CAD build for the part. Positions are in the model's coordinates, mm. Give positions to 0.01 mm unless a question says otherwise; leave off trailing zeros. Loops run counter-clockwise (first coordinate to the right, second up) from the corner with the lowest first, then second, coordinate; pieces in that order, holes last.
Item 1: Saw through at D-D on z = 5.5. Give the cut face in (x, y).
Item 2: Mould opens along X. For faces 1 (the flat face through (0, 0, -12)), 2 (the flat face through (-9.525, 2, -13)), 3 (the cylindrical face through (0.28, 1.9, -27.54)) say: released by +X, released by -X, zero draft, split by the parting line, or undercut.
Item 3: Saw through at C-C on z = 1. Give the cut face in (x, y), plus the area to 3 significant figures.
Item 4: Saw through at B-B on y = 2.95. Give the cut face in (x, z) (3 decimals), plus the area to 3 significant figures.
Item 5: Probe probe 1 along Z at (x, y) = (0, 1) (3 decimals); probe 2 along X at (y, z) = (2.75, -25) (3 decimals); probe 3 along X at (y, z) = (0.65, -1.5) (3 decimals). List the from-to ranges inside material, lowest first.
Item 6: Saw through at A-A on x = 0. Give the cut face in (y, z) (3 decimals), plus the area to 3 significant figures.
Item 7: Drop flat-ended pins along their axis: P1, Ø3.5, axis at x = 0, z = -25.4, coming from the +Y side; P2, Ø8, axis at x = -1.5, z = -19, coming from the -Y side. Give the stop position or say it passes through.
Autodesk Inventor part; units mm, degrees
ref_plane "YZ Plane" through (0, 0, 0) normal (1, 0, 0) x (0, 1, 0)
ref_plane "XZ Plane" through (0, 0, 0) normal (0, 1, 0) x (-1, 0, 0)
ref_plane "XY Plane" through (0, 0, 0) normal (0, 0, 1) x (1, 0, 0)
sketch "Sketch1" plane through (0, 0, 0) normal (0, 1, 0) x (-1, 0, 0)
  circle A0 centre (0, 0) radius 2.159
  circle A1 centre (0, -25.4) radius 2.159
  line L0 (0, 0) -> (0, -25.4) construction
  line L1 (-9.525, 0) -> (-9.525, -25.4)
  line L2 (9.525, -25.4) -> (9.525, 0)
  arc A2 (9.525, 0) -> (-9.525, 0) centre (0, 0) ccw
  arc A3 (-9.525, -25.4) -> (9.525, -25.4) centre (0, -25.4) ccw
  point P0 (0, -12.7)
  dimension "d0" = 4.318
  dimension "d2" = 25.4
  dimension "d3" = 19.05
extrude "Extrusion1" add sketch "Sketch1" along normal blind 3.861
properties part number "Small Motor Spacer" material "PET Plastic"
Results below:
1. outline: (-7.78, 0) - (7.78, 0) - (7.78, 3.86) - (-7.78, 3.86) - close
2. face 1: zero draft
2. face 2: released by -X
2. face 3: undercut
3. outline: (-9.47, 0) - (-1.91, 0) - (-1.91, 3.86) - (-9.47, 3.86) - close; (1.91, 0) - (9.47, 0) - (9.47, 3.86) - (1.91, 3.86) - close
3. area: 58.4 mm2
4. outline: (-9.525, -25.4) arc R9.525 ccw to (9.525, -25.4) - (9.525, 0) arc R9.525 ccw to (-9.525, 0) - close; hole circle Ø4.318 at (0, -25.4); hole circle Ø4.318 at (0, 0)
4. area: 740 mm2
5. probe 1: z = -34.925 to -27.559, -23.241 to -2.159, 2.159 to 9.525
5. probe 2: x = -9.525 to -2.122, 2.122 to 9.525
5. probe 3: x = -9.525 to -1.553, 1.553 to 9.525
6. outline: (0, -34.925) - (3.861, -34.925) - (3.861, -27.559) - (0, -27.559) - close; (0, -23.241) - (3.861, -23.241) - (3.861, -2.159) - (0, -2.159) - close; (0, 2.159) - (3.861, 2.159) - (3.861, 9.525) - (0, 9.525) - close
6. area: 138 mm2
7. P1: passes through
7. P2: stops at y = 0
